Part print with two shaded views. Sizes in mm from the minimum x, y, z corner. A direction names the side the tool comes from. Round coordinates to 2 decimals unless told otherwise and drop trailing zeros. Write each loop counter-clockwise with the first axis right and the second up, starting at its lowest first coordinate (ties: lowest second). Pieces come first, ordered by that corner, then holes. Notation, with made-up numbers: (57.25, 56) -> (114.25, 56) arc R26 cw to (114.25, 89) -> close; hole circle Ø4 at (-24, -37). An arc over 180 degrees is marked (long way). Put each result on its own line as item: value. Start each with the question number.
1. Drill centre lines: line 1 (Y direction, x = 7, z = 6.5); line 2 (Y direction, x = 83, z = 2.25); line 3 (X direction, y = 65, z = 6). Where is each one in solid material? Low to high. Write a range as from..to.
2. Flat gauge pins, fed straight in: P1, Ø3, axis at x = 72.5, y = 56, coming from the +Z side; P2, Ø2.5, axis at y = 4.5, z = 5, coming from the +X side; P3, Ø4, axis at y = 38, z = 6.5, coming from the +X side; P4, Ø4, axis at x = 5.5, z = 4.5, coming from the -Y side. Where does each tip first touch, or does it go through?
3. Saw through at C-C on y = 85.5. List the corners of the cut face in (x, z).
4. Saw through at A-A on z = 3.25. List the corners of the cut face in (x, y).
5. Saw through at B-B on x = 33.5. List the corners of the cut face in (y, z).
6. 3-axis set-ups, long thin cutter, end or side, ignore diameter. For the marked faces 1, 2, 3 and 4: which of +Z, -Z, +X, -X, +Y, -Y reach the whole face in a straight line?
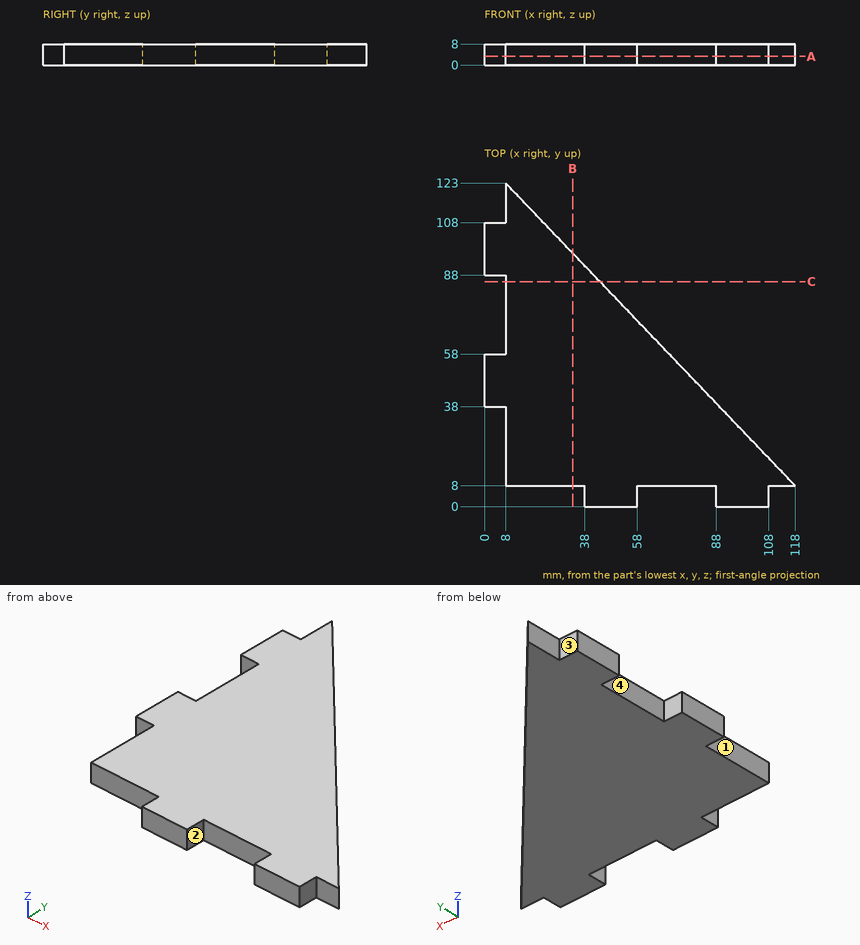
Return value:
1. line 1: y = 38..58, 88..108
1. line 2: y = 8..44.59
1. line 3: x = 8..63.48
2. P1: stops at z = 8
2. P2: stops at x = 108
2. P3: stops at x = 91.22
2. P4: stops at y = 38
3. outline: (8, 0) -> (43.87, 0) -> (43.87, 8) -> (8, 8) -> close
4. outline: (0, 38) -> (8, 38) -> (8, 8) -> (38, 8) -> (38, 0) -> (58, 0) -> (58, 8) -> (88, 8) -> (88, 0) -> (108, 0) -> (108, 8) -> (118, 8) -> (8, 123) -> (8, 108) -> (0, 108) -> (0, 88) -> (8, 88) -> (8, 58) -> (0, 58) -> close
5. outline: (8, 0) -> (96.34, 0) -> (96.34, 8) -> (8, 8) -> close
6. face 1: +Z, -Z, -X, -Y
6. face 2: +Z, -Z, -Y
6. face 3: +Z, -Z, -X, +Y
6. face 4: +Z, -Z, -X
